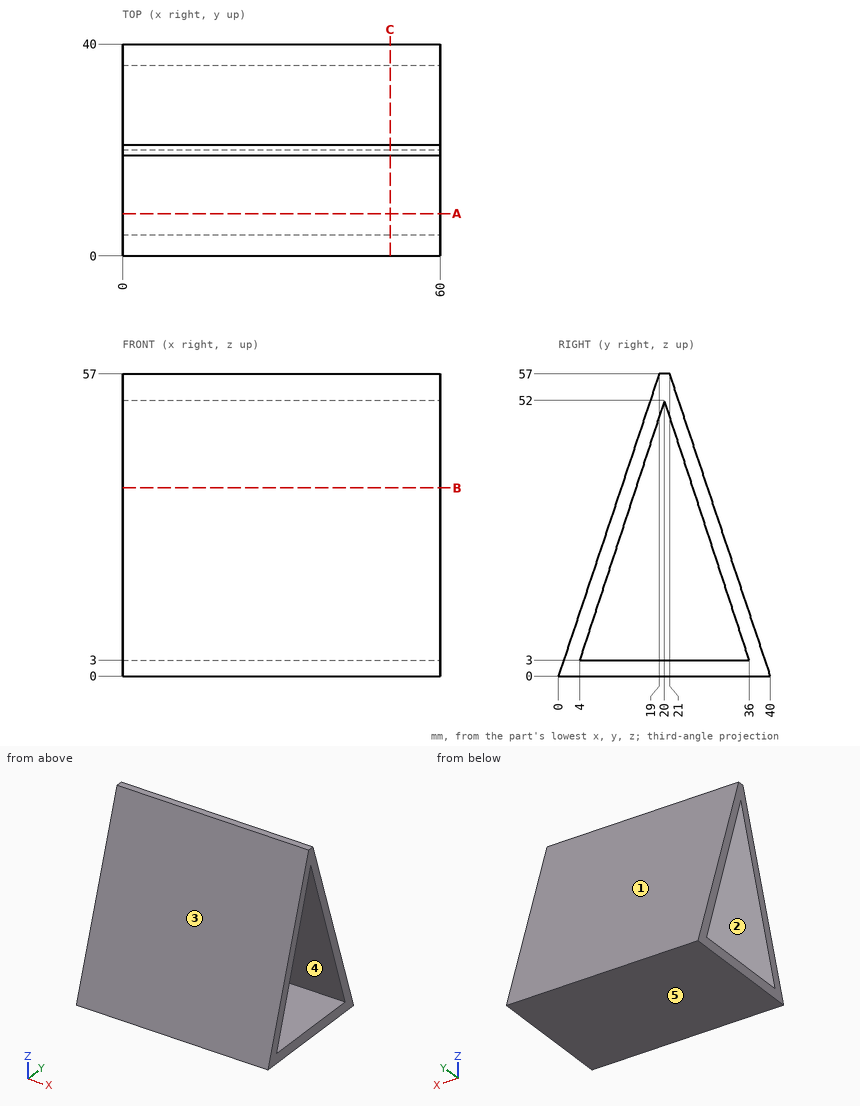
The drawing under review shows one solid part. Ordinate dimensions are in mm from its lowest x, y, z. A direction names the side the tool comes from. Round coordinates to 2 decimals unless told otherwise and drop trailing zeros. Loops run counter-clockwise (first coordinate to the right, second up) from the corner with the lowest first, then second, coordinate; pieces in that order, holes last. Notation, with made-up numbers: (50.25, 20) - (108.25, 20) arc R17 ccw to (108.25, 49) - close; hole circle Ø7 at (-30, 71.25). An arc over 180 degrees is marked (long way). Use a Markdown table: item, result. Add a question column.
Q1. For probe 1 along Y at (x, z) = (43, 49.5); probe 2 along Y at (x, z) = (27, 15.5); probe 3 along Y at (x, z) = (3, 55), list the stretches that pass through material, from the lowest coordinate up.
Q2. Machinability: for the marked faces 1 and 2, which of the approach directions +Z, -Z, +X, -X, +Y, -Y give a long, thin tool a straight path to every point of the face, cutting with its end or side? Answer none if there is none.
Q3. Add section A-A (y = 8). State the section outline as (x, z) points, plus the area to 3 significant figures.
Q4. Insertion check: pin 1 Ø1 at (x, z) = (8.5, 47.5) entering from +Y; pin 2 Ø5 at (x, z) = (45.5, 20.5) entering from +Y; pin 3 Ø10 at (y, z) = (31, 50.5) entering from -X. Each pin has a flat end and moves straight along its axis. Give the tip position at first contact, or say it passes through.
Q5. The part is to be moulded in two halves that separate along Z. For the marked faces 3, 4 and 5, say which applies: pulls with the +Z half, pulls with the -Z half, needs draft (parallel to the pull), parting line crosses it, or undercut.
Q6. Add section B-B (z = 35.5). State the section outline as (x, y) points, plus the area to 3 significant figures.
Q7. Add section C-C (x = 50.5). State the section outline as (y, z) points.
Worked answers:
| question | item | result |
|---|---|---|
| 1 | probe 1 | 16.5 to 19.18, 20.82 to 23.5 |
| 1 | probe 2 | 5.17 to 8.08, 31.92 to 34.83 |
| 1 | probe 3 | 18.33 to 21.67 |
| 2 | face 1 | +Z, +X, -X, +Y |
| 2 | face 2 | +X, -X |
| 3 | outline | (0, 0) - (60, 0) - (60, 3) - (0, 3) - close; (0, 15.25) - (60, 15.25) - (60, 24) - (0, 24) - close |
| 3 | area | 705 mm² |
| 4 | pin 1 | y = 24.33 |
| 4 | pin 2 | y = 34 |
| 4 | pin 3 | through |
| 5 | face 3 | pulls with the +Z half |
| 5 | face 4 | undercut |
| 5 | face 5 | pulls with the -Z half |
| 6 | outline | (0, 11.83) - (60, 11.83) - (60, 14.61) - (0, 14.61) - close; (0, 25.39) - (60, 25.39) - (60, 28.17) - (0, 28.17) - close |
| 6 | area | 333 mm² |
| 7 | outline | (0, 0) - (40, 0) - (21, 57) - (19, 57) - close; hole (4, 3) - (36, 3) - (20, 52) - close |
